Part model, mm, in its own coordinate system. Face numbers are marked on the shaded views. A direction names the side the tool comes from. Round coordinates to 2 decimals unless told otherwise and drop trailing zeros. Write each loop counter-clockwise with the first axis right and the second up, starting at its lowest first coordinate (ties: lowest second). Pieces come first, ordered by that corner, then holes. Notation, with made-up numbers: M 58.25,32.5 L 103.25,32.5 A24 ccw 103.25,49.5 Z; hole C 70.25,76.5 d5. An arc over 180 degrees is marked long. Answer as a JSON object with one key per item and string values. Group by question number.
1. Two-plate mould, pull along Y, no slides. Class the marked faces 3, 4, 5 and 6: +Y half, -Y half, draft (parallel to the pull), parting line (faces both ways), or undercut.
2. Band-saw the part on A-A, the plane x = 15.5. Write the cut outline in (y, z).
3. Drill centre lines: line 1 (X direction, y = 6, z = 2.25); line 2 (Y direction, x = -14.5, z = 11). Where is each one in solid material? Low to high. Write a range as from..to.
4. Drop a flat-ended pin along its axis: pin 1 (3 mm diameter, centred on x = 49.58, y = 62.33, fed in from -Z). Give the stop position or say it passes through.
5. Which spindle directions (+Z, -Z, +X, -X, +Y, -Y) get a long thin tool onto all of the face, cutting with end or side? Do the marked faces 1 and 2. Say none if no direction does.
6. Band-saw the part on C-C, the plane z = 15.75. Count the separate pieces of the cut face and the enclosed holes in it, plus the area to 3 significant figures.
7. Band-saw the part on B-B, the plane y = 23.5. Write the cut outline in (x, z), plus the area to 3 significant figures.
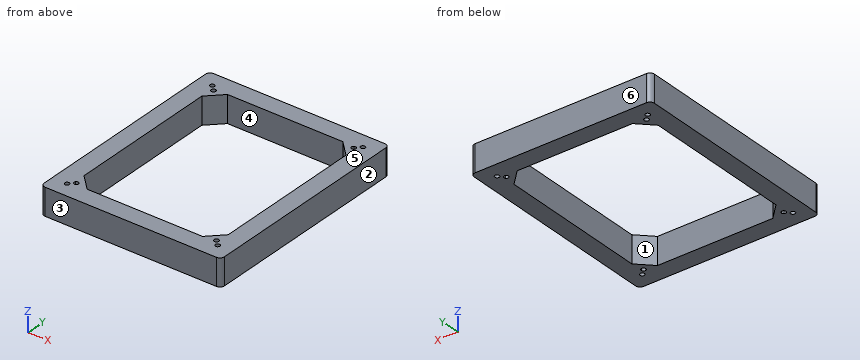
from build123d import *

# Parameters (mm, degrees)
F0_R     = 1.5875
F1_DEPTH = 19.05


with BuildPart() as f1:
    # F0 (on Top) → F1 (new body)
    with BuildSketch(Plane.XY):
        with BuildLine():
            Line((60.531797, 76.456334), (-60.118203, 76.456334))
            ThreePointArc((-60.118203, 76.456334), (-62.363267, 75.526399), (-63.293203, 73.281334))
            Line((-63.293203, 73.281334), (-63.293203, -72.768666))
            ThreePointArc((-63.293203, -72.768666), (-62.363267, -75.01373), (-60.118203, -75.943666))
            Line((-60.118203, -75.943666), (60.531797, -75.943666))
            ThreePointArc((60.531797, -75.943666), (62.776861, -75.01373), (63.706797, -72.768666))
            Line((63.706797, -72.768666), (63.706797, 73.281334))
            ThreePointArc((63.706797, 73.281334), (62.776861, 75.526399), (60.531797, 76.456334))
        make_face()
        with BuildLine():
            ThreePointArc((-56.943203, 66.931334), (-56.013267, 69.176399), (-53.768203, 70.106334))
            Line((-53.768203, 70.106334), (54.181797, 70.106334))
            ThreePointArc((54.181797, 70.106334), (56.426861, 69.176399), (57.356797, 66.931334))
            Line((57.356797, 66.931334), (57.356797, -66.418666))
            ThreePointArc((57.356797, -66.418666), (56.426861, -68.66373), (54.181797, -69.593666))
            Line((54.181797, -69.593666), (-53.768203, -69.593666))
            ThreePointArc((-53.768203, -69.593666), (-56.013267, -68.66373), (-56.943203, -66.418666))
            Line((-56.943203, -66.418666), (-56.943203, 66.931334))
        make_face(mode=Mode.SUBTRACT)
        with BuildLine():
            Line((54.181797, 70.106334), (-53.768203, 70.106334))
            ThreePointArc((-53.768203, 70.106334), (-56.013267, 69.176399), (-56.943203, 66.931334))
            Line((-56.943203, 66.931334), (-56.943203, -66.418666))
            ThreePointArc((-56.943203, -66.418666), (-56.013267, -68.66373), (-53.768203, -69.593666))
            Line((-53.768203, -69.593666), (54.181797, -69.593666))
            ThreePointArc((54.181797, -69.593666), (56.426861, -68.66373), (57.356797, -66.418666))
            Line((57.356797, -66.418666), (57.356797, 66.931334))
            ThreePointArc((57.356797, 66.931334), (56.426861, 69.176399), (54.181797, 70.106334))
        make_face()
        with Locations((-52.834257, -65.484719)):
            Circle(F0_R, mode=Mode.SUBTRACT)
        with BuildLine():
            ThreePointArc((-48.268948, 63.640233), (-47.847518, 63.727175), (-47.418203, 63.756334))
            Line((-47.418203, 63.756334), (-40.433203, 63.756334))
            Line((-40.433203, 63.756334), (40.846797, 63.756334))
            Line((40.846797, 63.756334), (47.831797, 63.756334))
            ThreePointArc((47.831797, 63.756334), (48.261112, 63.727175), (48.682541, 63.640233))
            ThreePointArc((48.682541, 63.640233), (50.321889, 63.738981), (51.171406, 62.333443))
            ThreePointArc((51.171406, 62.333443), (51.099604, 61.861412), (50.890695, 61.432079))
            ThreePointArc((50.890695, 61.432079), (50.977637, 61.01065), (51.006797, 60.581334))
            Line((51.006797, 60.581334), (51.006797, 53.596334))
            Line((51.006797, 53.596334), (51.006797, -53.083666))
            Line((51.006797, -53.083666), (51.006797, -60.698242))
            ThreePointArc((51.006797, -60.698242), (51.000133, -60.882306), (50.980177, -61.065405))
            ThreePointArc((50.980177, -61.065405), (51.122856, -61.431175), (51.171406, -61.820774))
            ThreePointArc((51.171406, -61.820774), (50.39662, -63.184465), (48.828536, -63.217046))
            ThreePointArc((48.828536, -63.217046), (48.645437, -63.237002), (48.461374, -63.243666))
            Line((48.461374, -63.243666), (40.846797, -63.243666))
            Line((40.846797, -63.243666), (-40.433203, -63.243666))
            Line((-40.433203, -63.243666), (-47.418203, -63.243666))
            ThreePointArc((-47.418203, -63.243666), (-47.847518, -63.214506), (-48.268948, -63.127564))
            ThreePointArc((-48.268948, -63.127564), (-50.292844, -62.943306), (-50.477102, -60.91941))
            ThreePointArc((-50.477102, -60.91941), (-50.564044, -60.497981), (-50.593203, -60.068666))
            Line((-50.593203, -60.068666), (-50.593203, -53.083666))
            Line((-50.593203, -53.083666), (-50.593203, 53.596334))
            Line((-50.593203, 53.596334), (-50.593203, 60.581334))
            ThreePointArc((-50.593203, 60.581334), (-50.564044, 61.01065), (-50.477102, 61.432079))
            ThreePointArc((-50.477102, 61.432079), (-50.292844, 63.455975), (-48.268948, 63.640233))
        make_face(mode=Mode.SUBTRACT)
        with Locations((53.24785, -65.484719)):
            Circle(F0_R, mode=Mode.SUBTRACT)
        with Locations((-52.834257, 65.997388)):
            Circle(F0_R, mode=Mode.SUBTRACT)
        with Locations((53.24785, 65.997388)):
            Circle(F0_R, mode=Mode.SUBTRACT)
        with BuildLine():
            Line((-40.433203, 63.756334), (-47.418203, 63.756334))
            ThreePointArc((-47.418203, 63.756334), (-47.847518, 63.727175), (-48.268948, 63.640233))
            ThreePointArc((-48.268948, 63.640233), (-47.764774, 63.071427), (-47.582812, 62.333443))
            ThreePointArc((-47.582812, 62.333443), (-48.69828, 60.817745), (-50.477102, 61.432079))
            ThreePointArc((-50.477102, 61.432079), (-50.564044, 61.01065), (-50.593203, 60.581334))
            Line((-50.593203, 60.581334), (-50.593203, 53.596334))
            Line((-50.593203, 53.596334), (-40.433203, 63.756334))
        make_face()
        with BuildLine():
            Line((47.831797, 63.756334), (40.846797, 63.756334))
            Line((40.846797, 63.756334), (51.006797, 53.596334))
            Line((51.006797, 53.596334), (51.006797, 60.581334))
            ThreePointArc((51.006797, 60.581334), (50.977637, 61.01065), (50.890695, 61.432079))
            ThreePointArc((50.890695, 61.432079), (48.461374, 61.210911), (48.682541, 63.640233))
            ThreePointArc((48.682541, 63.640233), (48.261112, 63.727175), (47.831797, 63.756334))
        make_face()
        with BuildLine():
            Line((51.006797, -60.698242), (51.006797, -53.083666))
            Line((51.006797, -53.083666), (40.846797, -63.243666))
            Line((40.846797, -63.243666), (48.461374, -63.243666))
            ThreePointArc((48.461374, -63.243666), (48.645437, -63.237002), (48.828536, -63.217046))
            ThreePointArc((48.828536, -63.217046), (48.461374, -60.698242), (50.980177, -61.065405))
            ThreePointArc((50.980177, -61.065405), (51.000133, -60.882306), (51.006797, -60.698242))
        make_face()
        with BuildLine():
            Line((-40.433203, -63.243666), (-50.593203, -53.083666))
            Line((-50.593203, -53.083666), (-50.593203, -60.068666))
            ThreePointArc((-50.593203, -60.068666), (-50.564044, -60.497981), (-50.477102, -60.91941))
            ThreePointArc((-50.477102, -60.91941), (-48.69828, -60.305076), (-47.582812, -61.820774))
            ThreePointArc((-47.582812, -61.820774), (-47.764774, -62.558758), (-48.268948, -63.127564))
            ThreePointArc((-48.268948, -63.127564), (-47.847518, -63.214506), (-47.418203, -63.243666))
            Line((-47.418203, -63.243666), (-40.433203, -63.243666))
        make_face()
    extrude(amount=F1_DEPTH)


solid = f1.part
Worked answers:
{
 "1": {"face 3": "-Y half", "face 4": "undercut", "face 5": "draft", "face 6": "+Y half"},
 "2": {"outline": "M -75.94,0 L -63.24,0 L -63.24,19.05 L -75.94,19.05 Z; M 63.76,0 L 76.46,0 L 76.46,19.05 L 63.76,19.05 Z"},
 "3": {"line 1": "x = -63.29..-50.59, 51.01..63.71", "line 2": "y = -75.94..-63.24, 63.76..76.46"},
 "4": {"pin 1": "passes through"},
 "5": {"face 1": "+Z, -Z", "face 2": "+Z, -Z, +X, +Y, -Y"},
 "6": {"separate pieces": "1", "enclosed holes": "9", "area": "6,590 mm^2"},
 "7": {"outline": "M -63.29,0 L -50.59,0 L -50.59,19.05 L -63.29,19.05 Z; M 51.01,0 L 63.71,0 L 63.71,19.05 L 51.01,19.05 Z", "area": "484 mm^2"}
}
